Check sheet for the modelled part. Datum: model origin and axes. Units: mm. Face numbers are marked on the shaded views. A direction names the side the tool comes from. Coordinates: 2 decimals unless noted, no trailing zeros. Order: outer loops, then holes, each group sorted by start corner. A loop starts at its lowest first (then second) coordinate and runs counter-clockwise, first axis right, second up.
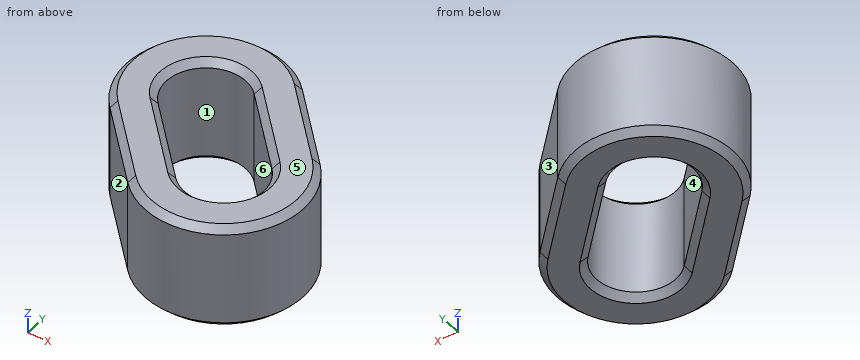
from build123d import *

# Parameters (mm, degrees)
BOSS_EXTRUDE1_DEPTH = 8
CHAMFER1_SIZE       = 0.5


with BuildPart() as part:
    # Sketch1 → Boss-Extrude1 (new body)
    with BuildSketch(Plane.XY):
        with BuildLine():
            Line((69.900235992, 117.557359313), (75.118684037, 112.338911268))
            ThreePointArc((75.118684037, 112.338911268), (83.603965411, 112.338911268), (83.603965411, 120.824192642))
            Line((83.603965411, 120.824192642), (78.385517366, 126.042640687))
            ThreePointArc((78.385517366, 126.042640687), (69.900235992, 126.042640687), (69.900235992, 117.557359313))
        make_face()
        with BuildLine():
            Line((72.021556335, 119.678679656), (77.24000438, 114.460231611))
            ThreePointArc((77.24000438, 114.460231611), (81.482645068, 114.460231611), (81.482645068, 118.702872298))
            Line((81.482645068, 118.702872298), (76.264197022, 123.921320344))
            ThreePointArc((76.264197022, 123.921320344), (72.021556335, 123.921320344), (72.021556335, 119.678679656))
        make_face(mode=Mode.SUBTRACT)
    extrude(amount=BOSS_EXTRUDE1_DEPTH)

    # Chamfer1
    chamfer1_edges = [part.edges().sort_by_distance(p)[0] for p in [
        (83.603965411, 112.338911268, 8),
        (80.994741388, 123.433416665, 8),
        (72.021556335, 123.921320344, 0),
        (74.630780358, 117.069455634, 0),
        (81.482645068, 114.460231611, 0),
        (78.873421045, 121.312096321, 0),
        (72.021556335, 123.921320344, 8),
        (74.630780358, 117.069455634, 8),
        (81.482645068, 114.460231611, 8),
        (78.873421045, 121.312096321, 8),
        (69.900235992, 126.042640687, 8),
        (80.994741388, 123.433416665, 0),
        (83.603965411, 112.338911268, 0),
        (72.509460014, 114.94813529, 0),
        (69.900235992, 126.042640687, 0),
        (72.509460014, 114.94813529, 8),
    ]]
    chamfer(chamfer1_edges, length=CHAMFER1_SIZE)


solid = part.part
(1) Tool access check on the marked faces 5 and 6. Record the directions out of +Z, -Z, +X, -X, +Y, -Y that give a thin tool (end or side, any length) a straight path to the whole face; none if there is none.
Filled in:
face 5: +Z, +X, -X, +Y, -Y
face 6: +Z, -Z
(2) Go/stop test with flat-tipped pins: P1, Ø4, axis at x = 71, y = 121.5, coming from the -Z side; P2, Ø1, axis at y = 121, z = 7, coming from the +X side. Record where each tip stops, or that it passes through.
Filled in:
P1: stops at z = 0
P2: stops at x = 83.91
(3) Release check for a two-part mould opening along Y. For the marked faces 1, 2, 3 and 4 record: +Y half, -Y half, draft (parallel to the pull), parting line (faces both ways), or undercut.
Filled in:
face 1: undercut
face 2: -Y half
face 3: +Y half
face 4: undercut
(4) Cross-section at B-B (y = 121.8). Enter the section's corners in (x, z), and give its area (3 significant figures).
Filled in:
outline: (68.14, 0.5) - (68.64, 0) - (70.64, 0) - (71.14, 0.5) - (71.14, 7.5) - (70.64, 8) - (68.64, 8) - (68.14, 7.5) - close; (78.39, 0.5) - (79.09, 0) - (81.92, 0) - (82.63, 0.5) - (82.63, 7.5) - (81.92, 8) - (79.09, 8) - (78.39, 7.5) - close
area: 56.7 mm2
(5) Thickness scan on probe 1 along Y at (x, z) = (78, 7); probe 2 along Y at (x, z) = (72.5, 2.25); probe 3 along X at (y, z) = (115.25, 3.5). Record the ranges inside material, lowest first.
Filled in:
probe 1: y = 110.74 to 113.91, 122.19 to 126.4
probe 2: y = 114.96 to 119.2, 124.31 to 127.57
probe 3: x = 72.21 to 76.45, 82.05 to 85.21
